Could you check a few things on this model? Use its own coordinates, in mm. Face numbers are marked on the shaded views. Round coordinates to 2 decimals unless told otherwise and drop trailing zeros. Loops run counter-clockwise (first coordinate to the right, second up) from the corner with the lowest first, then second, coordinate; pieces in that order, holes last. Notation, with made-up numbers: (-9, 56.5) -> (21, 56.5) arc R20 cw to (21, 61.5) -> close; hole circle Ø6 at (36.25, 52.5). An arc over 180 degrees is marked (long way). One line per item, written item: value.
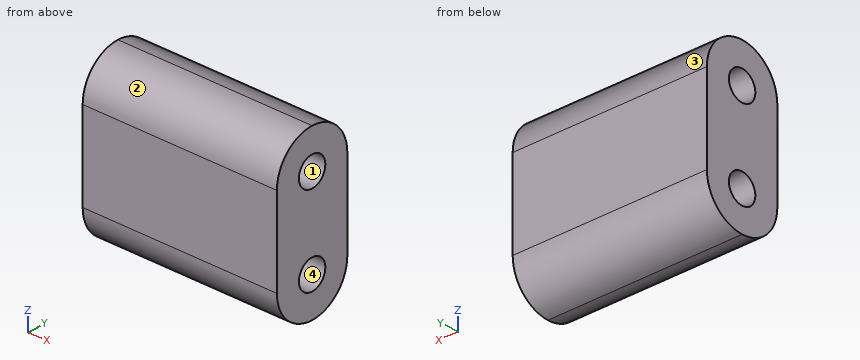
```python
from build123d import *

# Parameters (mm, degrees)
SKETCH1_W           = 12.7
SKETCH1_H           = 10.795
BOSS_EXTRUDE1_DEPTH = 5.08
CUT_EXTRUDE1_REACH  = 19.425
SKETCH2_R           = 0.9525
FILLET1_R           = 2.54


with BuildPart() as part:
    # Sketch1 → Boss-Extrude1 (new body)
    with BuildSketch(Plane(origin=(0, 0, 0), x_dir=(1, 0, 0), z_dir=(0, 1, 0))):
        with Locations((6.35, 5.3975)):
            Rectangle(SKETCH1_W, SKETCH1_H)
    extrude(amount=BOSS_EXTRUDE1_DEPTH)

    # Sketch2 → Cut-Extrude1 (cut, up to next)
    with BuildSketch(Plane(origin=(12.7, 0, 0), x_dir=(0, 0, -1), z_dir=(1, 0, 0)), mode=Mode.PRIVATE) as cut_extrude1_sk1:
        with Locations((2.54, 2.54)):
            Circle(SKETCH2_R)
    cut_extrude1_tool1 = extrude(cut_extrude1_sk1.sketch, amount=-CUT_EXTRUDE1_REACH, mode=Mode.PRIVATE) & part.part
    # Sketch2 → Cut-Extrude1 (cut, up to next)
    with BuildSketch(Plane(origin=(12.7, 0, 0), x_dir=(0, 0, -1), z_dir=(1, 0, 0)), mode=Mode.PRIVATE) as cut_extrude1_sk2:
        with Locations((8.255, 2.54)):
            Circle(SKETCH2_R)
    cut_extrude1_tool2 = extrude(cut_extrude1_sk2.sketch, amount=-CUT_EXTRUDE1_REACH, mode=Mode.PRIVATE) & part.part
    add(cut_extrude1_tool1.solids().sort_by_distance((12.7, 2.54, -2.54))[0], mode=Mode.SUBTRACT)
    add(cut_extrude1_tool2.solids().sort_by_distance((12.7, 2.54, -8.255))[0], mode=Mode.SUBTRACT)

    # Fillet1
    fillet1_edges = [part.edges().sort_by_distance(p)[0] for p in [
        (6.35, 0, -10.795),
        (6.35, 5.08, -10.795),
        (6.35, 0, 0),
        (6.35, 5.08, 0),
    ]]
    fillet(fillet1_edges, radius=FILLET1_R - 0.0001)  # a hair under: the kernel refuses the full size


solid = part.part
```
Item 1: I need wall thicknesses on line 1 (Y direction, x = 9, z = -2.5); line 2 (Z direction, x = 4.75, y = 2.85); line 3 (Y direction, x = 1, z = -1.75). Which ranges of each line are inside material? Lowest first, please. Write a range as from..to.
Output:
line 1: y = 0..1.59, 3.49..5.08
line 2: z = -10.78..-9.16, -7.35..-3.44, -1.64..-0.02
line 3: y = 0.13..2.01, 3.07..4.95
Item 2: If we section it at B-B on y = 2.85: List the corners of the cut face in (x, z) for me, plus the area to 3 significant figures.
Output:
outline: (0, -10.78) -> (12.7, -10.78) -> (12.7, -9.16) -> (0, -9.16) -> close; (0, -7.35) -> (12.7, -7.35) -> (12.7, -3.44) -> (0, -3.44) -> close; (0, -1.64) -> (12.7, -1.64) -> (12.7, -0.02) -> (0, -0.02) -> close
area: 90.9 mm²
Item 3: If we section it at C-C on z = -1.75: List the corners of the cut face in (x, y) for me, plus the area to 3 significant figures.
Output:
outline: (0, 0.13) -> (12.7, 0.13) -> (12.7, 2.01) -> (0, 2.01) -> close; (0, 3.07) -> (12.7, 3.07) -> (12.7, 4.95) -> (0, 4.95) -> close
area: 47.8 mm²
Item 4: If we section it at D-D on y = 1.8: List the corners of the cut face in (x, z) for me.
Output:
outline: (0, -10.68) -> (12.7, -10.68) -> (12.7, -8.85) -> (0, -8.85) -> close; (0, -7.66) -> (12.7, -7.66) -> (12.7, -3.14) -> (0, -3.14) -> close; (0, -1.94) -> (12.7, -1.94) -> (12.7, -0.11) -> (0, -0.11) -> close
Item 5: If we mould it in two halves opening along Y, with no side actions, what happens to the marked faces 1, 2, 3 and 4? For each: released by +Y, released by -Y, zero draft, split by the parting line, or undercut.
Output:
face 1: undercut
face 2: released by -Y
face 3: released by +Y
face 4: undercut
Item 6: If we section it at A-A on x = 10: Count the separate pieces of the cut face and the enclosed holes in it, plus the area to 3 significant figures.
Output:
separate pieces: 1
enclosed holes: 2
area: 43.6 mm²
